Check sheet for the modelled part. Datum: model origin and axes. Units: mm. Round coordinates to 2 decimals unless told otherwise and drop trailing zeros. Answer in a Markdown table with one row per item.
from build123d import *

# Parameters (mm, degrees)
BOSS_EXTRUDE1_DEPTH = 5
SKETCH2_R           = 2.5
SKETCH2_W           = 35
SKETCH2_H           = 75
CUT_EXTRUDE1_DEPTH  = 10
SKETCH4_R           = 2
CUT_EXTRUDE3_DEPTH  = 10
SKETCH5_R           = 2.5
CUT_EXTRUDE4_DEPTH  = 10


with BuildPart() as part:
    # Sketch1 → Boss-Extrude1 (new body)
    with BuildSketch(Plane.XY):
        with BuildLine():
            Line((77, 150.635083269), (106.477021815, 150.635083269))
            ThreePointArc((106.477021815, 150.635083269), (73.792570992, 172.830527842), (35.06273753, 180.635083269))
            Line((35.06273753, 180.635083269), (-264.93726247, 180.635083269))
            ThreePointArc((-264.93726247, 180.635083269), (-303.667095932, 172.830527842), (-336.351546756, 150.635083269))
            Line((-336.351546756, 150.635083269), (-306.874524941, 150.635083269))
            Line((-306.874524941, 150.635083269), (-306.874524941, 10.635083269))
            Line((-306.874524941, 10.635083269), (-336.351546756, 10.635083269))
            ThreePointArc((-336.351546756, 10.635083269), (-303.667095932, -11.560361304), (-264.93726247, -19.364916731))
            Line((-264.93726247, -19.364916731), (35.06273753, -19.364916731))
            ThreePointArc((35.06273753, -19.364916731), (73.792570992, -11.560361304), (106.477021815, 10.635083269))
            Line((106.477021815, 10.635083269), (77, 10.635083269))
            Line((77, 10.635083269), (77, 150.635083269))
        make_face()
    extrude(amount=-BOSS_EXTRUDE1_DEPTH)

    # Sketch2 → Cut-Extrude1 (cut)
    with BuildSketch(Plane(origin=(0, 0, -5), x_dir=(-1, 0, 0), z_dir=(0, 0, -1))):
        with Locations((301.874524941, 106.135083269)):
            Circle(SKETCH2_R)
        with Locations(Location((301.874524941, 55.135083269, 0), (0, 0, 180))):
            Circle(SKETCH2_R)
        with Locations((-72, 55.135083269)):
            Circle(SKETCH2_R)
        with Locations(Location((-72, 106.135083269, 0), (0, 0, 180))):
            Circle(SKETCH2_R)
        with Locations((219.374524941, 80.635083269)):
            Rectangle(SKETCH2_W, SKETCH2_H)
        with Locations((10.5, 80.635083269)):
            Rectangle(SKETCH2_W, SKETCH2_H)
    extrude(amount=-CUT_EXTRUDE1_DEPTH, mode=Mode.SUBTRACT)

    # Sketch4 → Cut-Extrude3 (cut)
    with BuildSketch(Plane(origin=(0, 0, -5), x_dir=(-1, 0, 0), z_dir=(0, 0, -1))):
        with Locations((46, 64.695083269)):
            Circle(SKETCH4_R)
        with Locations((46, 96.695083269)):
            Circle(SKETCH4_R)
        with Locations((78, 64.695083269)):
            Circle(SKETCH4_R)
        with Locations((78, 96.695083269)):
            Circle(SKETCH4_R)
        with Locations(Location((151.874524941, 64.695083269, 0), (0, 0, 180))):
            Circle(SKETCH4_R)
        with Locations(Location((183.874524941, 64.695083269, 0), (0, 0, 180))):
            Circle(SKETCH4_R)
        with Locations(Location((183.874524941, 96.695083269, 0), (0, 0, 180))):
            Circle(SKETCH4_R)
        with Locations(Location((151.874524941, 96.695083269, 0), (0, 0, 180))):
            Circle(SKETCH4_R)
    extrude(amount=-CUT_EXTRUDE3_DEPTH, mode=Mode.SUBTRACT)

    # Sketch5 → Cut-Extrude4 (cut)
    with BuildSketch(Plane(origin=(0, 0, -5), x_dir=(-1, 0, 0), z_dir=(0, 0, -1))):
        with Locations((94.63726247, 168.635083269)):
            Circle(SKETCH5_R)
        with Locations((135.23726247, 168.635083269)):
            Circle(SKETCH5_R)
        with Locations(Location((94.63726247, -7.364916731, 0), (0, 0, 180))):
            Circle(SKETCH5_R)
        with Locations(Location((135.23726247, -7.364916731, 0), (0, 0, 180))):
            Circle(SKETCH5_R)
    extrude(amount=-CUT_EXTRUDE4_DEPTH, mode=Mode.SUBTRACT)


solid = part.part
Item 1: Scan lines: line 1 (Y direction, x = -78, z = -3.1); line 2 (X direction, y = 105.5, z = -0.5); line 3 (Y direction, x = -135, z = -1.45). Record each from-to range of solid material in increasing order. Write a range as [from, to].
Result sheet:
| item | result |
|---|---|
| line 1 | y = [-19.36, 62.7], [66.7, 94.7], [98.7, 180.64] |
| line 2 | x = [-306.87, -304.29], [-299.46, -236.87], [-201.87, -28], [7, 69.58], [74.42, 77] |
| line 3 | y = [-19.36, -9.85], [-4.88, 166.15], [171.12, 180.64] |
Item 2: Depth check by flat-ended pin: P1, Ø3, axis at y = 101, z = -1.5, coming from the -X side; P2, Ø2.5, axis at y = 73.5, z = -2.5, coming from the +X side; P3, Ø3.5, axis at x = -183.87, y = 64.7, coming from the -Z side; P4, Ø8, axis at x = -131.5, y = 139.5, coming from the +Z side. Enter the tip coordinate at first touch or a pass-through.
Result sheet:
| item | result |
|---|---|
| P1 | stops at x = -306.87 |
| P2 | stops at x = 77 |
| P3 | passes through |
| P4 | stops at z = 0 |
Item 3: Cross-section at A-A (z = -2.85). State how many separate pieces and enclosed holes the cut face has, and give its area (3 significant figures).
Result sheet:
| item | result |
|---|---|
| separate pieces | 1 |
| enclosed holes | 18 |
| area | 72,100 mm^2 |
